Read the model definition and answer for the solid it produces. Units are mm, in the model's axes. A direction names the side the tool comes from. Round coordinates to 2 decimals unless told otherwise and drop trailing zeros. Write each loop counter-clockwise with the first axis right and the second up, starting at its lowest first coordinate (ties: lowest second). Pieces come first, ordered by that corner, then holes. Notation, with made-up numbers: (-12, 5.25) - (3, 5.25) arc R37 ccw to (3, 44.25) - close; hole circle Ø7 at (76, -13). An arc over 180 degrees is marked (long way). Answer as CSV lines item,"result". Start each with the question number.
1) Find section D-D on y = 15.25. Determine the outline of the cut face in (x, z), then the cut area to 3 significant figures.
2) Which of the six approach directions +Z, -Z, +X, -X, +Y, -Y give full straight-line access (tool end or side, diameter ignored) to faces 5 (the flat face through (0, 16, 0)), 6 (the cylindrical face through (0, 7, 2)), 7 (the flat face through (0, 0, 0))?
3) Find section C-C on y = 2.75. Determine the outline of the cut face in (x, z).
4) For a pull along Z with two mould halves and no side action, classify faces 1 (the flat face through (2, 15, 2)), 2 (the cylindrical face through (3.233, 16.479, -1.341)), 3 (the flat face through (0.88, 17.01, 1.49)), 4 (the flat face through (-0.88, 17.01, -1.49)) as +Z half, -Z half, draft (parallel to the pull), parting line (faces both ways), or undercut.
5) Each of these flat-tipped pins is pushed along its axis until it touches: pin 1 (2 mm diameter, centred on y = 11.5, z = 1.5, fed in from -X); pin 2 (2 mm diameter, centred on y = 10, z = 2, fed in from -X); pin 3 (1 mm diameter, centred on x = -0.5, y = 14, fed in from -Z); pin 4 (2 mm diameter, centred on x = 1, z = -1, fed in from -Y). Where does it stop, or does it pass through?
6) Find section B-B on x = 1. Determine the outline of the cut face in (y, z), then the cut area to 3 significant figures.
7) Find section A-A on z = 0. Determine the outline of the cut face in (x, y), then the cut area to 3 significant figures.
8) Consider line 1 along Y through (x, z) = (1, -2); line 2 along Y through (x, z) = (0.5, 1.5); line 3 along Z through (x, y) = (-1, 16.25). Determine where each line is inside the solid, lowest interval first.
Autodesk Inventor part; units mm, degrees
ref_plane "YZ Plane" through (0, 0, 0) normal (1, 0, 0) x (0, 1, 0)
ref_plane "XZ Plane" through (0, 0, 0) normal (0, 1, 0) x (-1, 0, 0)
ref_plane "XY Plane" through (0, 0, 0) normal (0, 0, 1) x (1, 0, 0)
sketch "草圖1" plane through (0, 0, 0) normal (0, 1, 0) x (-1, 0, 0)
  circle A0 centre (0, 0) radius 2
  dimension "d0" = 4
extrude "擠出1" add sketch "草圖1" along normal blind 15
sketch "草圖2" plane through (0, 15, 0) normal (0, 1, 0) x (1, 0, 0)
  circle A0 centre (0, 0) radius 3.5
  dimension "d3" = 7
extrude "擠出2" add sketch "草圖2" along normal blind 3
sketch "草圖3" plane through (0, 18, 0) normal (0, 1, 0) x (1, 0, 0)
  circle A0 centre (0, 0) radius 2
  line L0 (0, 2) -> (1.7321, 1)
  line L1 (1.7321, 1) -> (1.7321, -1)
  line L2 (1.7321, -1) -> (0, -2)
  line L3 (0, -2) -> (-1.7321, -1)
  line L4 (-1.7321, -1) -> (-1.7321, 1)
  line L5 (-1.7321, 1) -> (0, 2)
extrude "擠出3" cut sketch "草圖3" against normal blind 2 contours L1 L2 L3 L4 L5 L0
thread "螺紋1"
properties part number "M4set_screw"
Check values:
1,outline,"circle Ø7 at (0, 0)"
1,area,"38.5 mm^2"
2,face 5,"+Y"
2,face 6,"-Y"
2,face 7,"+Z, -Z, +X, -X, -Y"
3,outline,"circle Ø4 at (0, 0)"
4,face 1,"draft"
4,face 2,"parting line"
4,face 3,"undercut"
4,face 4,"undercut"
5,pin 1,"stops at x = -1.94"
5,pin 2,"stops at x = -1.73"
5,pin 3,"stops at z = -2"
5,pin 4,"stops at y = 0"
6,outline,"(0, -1.73) - (15, -1.73) - (15, -3.35) - (18, -3.35) - (18, -1.42) - (16, -1.42) - (16, 1.42) - (18, 1.42) - (18, 3.35) - (15, 3.35) - (15, 1.73) - (0, 1.73) - close"
6,area,"66.4 mm^2"
7,outline,"(-3.5, 15) - (-2, 15) - (-2, 0) - (2, 0) - (2, 15) - (3.5, 15) - (3.5, 18) - (1.73, 18) - (1.73, 16) - (-1.73, 16) - (-1.73, 18) - (-3.5, 18) - close"
7,area,"74.1 mm^2"
8,line 1,"y = 15 to 18"
8,line 2,"y = 0 to 16"
8,line 3,"z = -3.35 to -1.42, 1.42 to 3.35"
